CAD build for the part. Positions are in the model's coordinates, mm. A direction names the side the tool comes from. Round coordinates to 2 decimals unless told otherwise and drop trailing zeros. Loops run counter-clockwise (first coordinate to the right, second up) from the corner with the lowest first, then second, coordinate; pieces in that order, holes last. Notation, with made-up numbers: M -16,-33.5 L 4,-33.5 A16 cw 4,-21.5 Z; hole C 37,34.5 d8. An arc over 180 degrees is marked long. Use a Markdown table: item, result. Add a question column.
(1) Two-plate mould, pull along Y, no slides. Class faces 5 (the face through (-82, 70, 2)), 6 (the face through (-8, 16.5, 3)), 7 (the face through (4, 55, 2)): released by +Y, released by -Y, zero draft, split by the parting line, or undercut.
(2) Which spindle directions (+Z, -Z, +X, -X, +Y, -Y) get a long thin tool onto all of the face, cutting with end or side? Do faces 1 (the face through (-80, 9, 2)), 2 (the face through (-13, 22.1, 3)), 3 (the face through (-8, 23.5, 3)), 4 (the face through (-77, 87.9, 3)). Say none if no direction does.
(3) Band-saw the part on B-B, the plane x = -65.5. Write the cut outline in (y, z).
(4) Wall check: L1, parallel to Y at x = -76, z = 2.75; L2, parallel to X at y = 23, z = 4.6; L3, parallel to Y at x = -71, z = 3.95. Give the ranges that are in metal, low to high.
(5) Band-saw the part on C-C, the plane y = 81. Write the cut outline in (x, z).
(6) Band-saw the part on A-A, the plane x = -8.5. Write the cut outline in (y, z).
(7) Flat gauge pins, fed straight in: P1, Ø2, axis at x = 2, z = 2, coming from the +Y side; P2, Ø1.5, axis at y = 23.5, z = 2.5, coming from the +X side; P3, Ø1.5, axis at x = -68, z = 3.5, coming from the -Y side; P4, Ø1.5, axis at y = 30, z = 3.5, coming from the -X side. Where does each tip first touch, or does it go through?
from build123d import *

# Parameters (mm, degrees)
ESQUISSE1_W             = 80
ESQUISSE1_H             = 110
BOSS_EXTRU_1_DEPTH      = 5
ENL_V_MAT_EXTRU_2_DEPTH = 137.106575888
ESQUISSE4_W             = 88
ESQUISSE4_H             = 30
BOSS_EXTRU_2_DEPTH      = 5


with BuildPart() as part:
    # Esquisse1 → Boss.-Extru.1 (new body)
    with BuildSketch(Plane.XY):
        with Locations((-40, 55)):
            Rectangle(ESQUISSE1_W, ESQUISSE1_H)
    extrude(amount=BOSS_EXTRU_1_DEPTH)

    # Esquisse3 → Enlèv. mat.-Extru.2 (cut, through all)
    with BuildSketch(Plane.XY.offset(5)):
        Polygon((-17, 87.9), (-10, 87.9), (-10, 86.5), (-6.8, 86.5), (-6.8, 87.9), (0, 87.9), (0, 92.1), (-6.8, 92.1), (-6.8, 93.5), (-10, 93.5), (-10, 92.1), (-17, 92.1), align=None)
        Polygon((-80, 92.1), (-80, 87.9), (-73.2, 87.9), (-73.2, 86.5), (-70, 86.5), (-70, 87.9), (-63, 87.9), (-63, 92.1), (-70, 92.1), (-70, 93.5), (-73.2, 93.5), (-73.2, 92.1), align=None)
        Polygon((-73.2, 22.1), (-80, 22.1), (-80, 17.9), (-73.2, 17.9), (-73.2, 16.5), (-70, 16.5), (-70, 17.9), (-63, 17.9), (-63, 22.1), (-70, 22.1), (-70, 23.5), (-73.2, 23.5), align=None)
        Polygon((0, 17.9), (0, 22.1), (-6.8, 22.1), (-6.8, 23.5), (-10, 23.5), (-10, 22.1), (-17, 22.1), (-17, 17.9), (-10, 17.9), (-10, 16.5), (-6.8, 16.5), (-6.8, 17.9), align=None)
    extrude(amount=-ENL_V_MAT_EXTRU_2_DEPTH, mode=Mode.SUBTRACT)

    # Esquisse4 → Boss.-Extru.2 (add)
    with BuildSketch(Plane(origin=(0, 0, 0), x_dir=(-1, 0, 0), z_dir=(0, 0, -1))):
        with Locations((40, 55)):
            Rectangle(ESQUISSE4_W, ESQUISSE4_H)
    extrude(amount=-BOSS_EXTRU_2_DEPTH)


solid = part.part
Return value:
| question | item | result |
|---|---|---|
| 1 | face 5 | released by +Y |
| 1 | face 6 | undercut |
| 1 | face 7 | zero draft |
| 2 | face 1 | +Z, -Z, -X, -Y |
| 2 | face 2 | +Z, -Z, +X |
| 2 | face 3 | +Z, -Z |
| 2 | face 4 | +Z, -Z, -X |
| 3 | outline | M 0,0 L 17.9,0 L 17.9,5 L 0,5 Z; M 22.1,0 L 87.9,0 L 87.9,5 L 22.1,5 Z; M 92.1,0 L 110,0 L 110,5 L 92.1,5 Z |
| 4 | L1 | 0 to 17.9, 22.1 to 87.9, 92.1 to 110 |
| 4 | L2 | -80 to -73.2, -70 to -10, -6.8 to 0 |
| 4 | L3 | 0 to 16.5, 23.5 to 86.5, 93.5 to 110 |
| 5 | outline | M -80,0 L 0,0 L 0,5 L -80,5 Z |
| 6 | outline | M 0,0 L 16.5,0 L 16.5,5 L 0,5 Z; M 23.5,0 L 86.5,0 L 86.5,5 L 23.5,5 Z; M 93.5,0 L 110,0 L 110,5 L 93.5,5 Z |
| 7 | P1 | y = 70 |
| 7 | P2 | x = 0 |
| 7 | P3 | y = 0 |
| 7 | P4 | x = -80 |
